Can you work these out from the drawing? Everything is in mm from the part's minimum corner. Round coordinates to 2 decimals unless told otherwise and drop trailing zeros. Loops run counter-clockwise (first coordinate to the right, second up) from the corner with the lowest first, then second, coordinate; pieces in that order, holes last. Notation, with made-up numbers: M -7.5,-25 L 16.5,-25 A18 ccw 16.5,-3 Z; hole C 78,-17.75 d9. An arc over 180 degrees is marked long. Return JSON: item names as keys, results as strings. Group by question number.
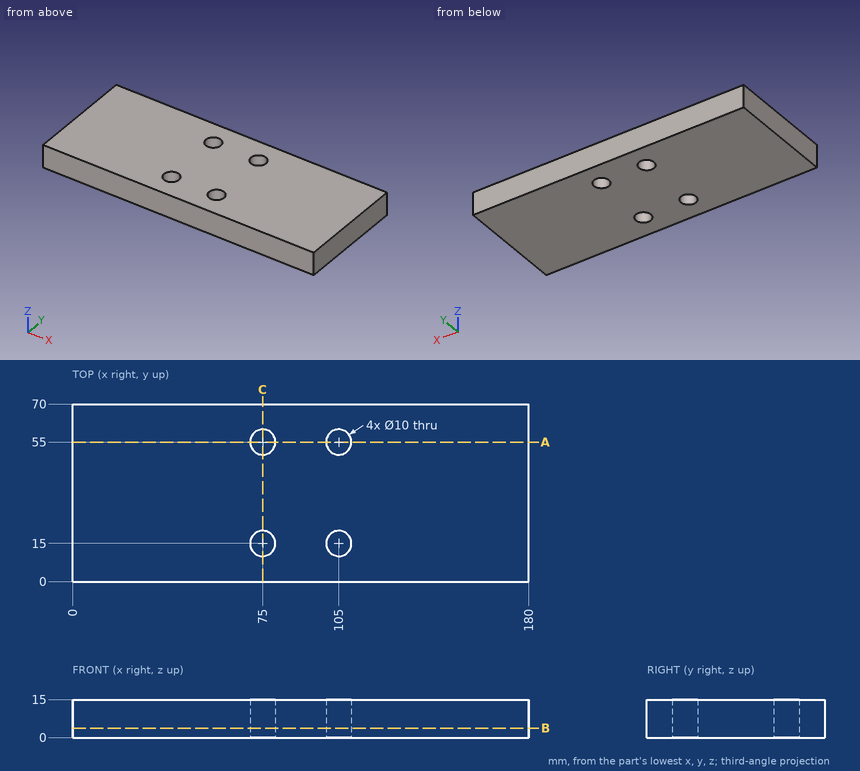
1. If we section it at B-B, the plane z = 3.75: Please give me the cut outline in (x, y), then the cut area to 3 significant figures.
2. If we section it at C-C, the plane x = 75: Please give me the cut outline in (y, z), then the cut area to 3 significant figures.
3. If we section it at A-A, the plane y = 55: Please give me the cut outline in (x, z), then the cut area to 3 significant figures.
4. I'm going to push a flat-ended pin straight in: pin 1 Ø4 at (x, y) = (130.5, 27) entering from -Z. Where does the tip first touch, or does it pass through?
5. I need wall thicknesses on probe 1 along Y at (x, z) = (105, 4.5); probe 2 along X at (y, z) = (54, 6.75). Which ranges of each line are inside material? Lowest first, please.
Geometry results:
{
 "1": {"outline": "M 0,0 L 180,0 L 180,70 L 0,70 Z; hole C 75,15 d10; hole C 75,55 d10; hole C 105,15 d10; hole C 105,55 d10", "area": "12,300 mm^2"},
 "2": {"outline": "M 0,0 L 10,0 L 10,15 L 0,15 Z; M 20,0 L 50,0 L 50,15 L 20,15 Z; M 60,0 L 70,0 L 70,15 L 60,15 Z", "area": "750 mm^2"},
 "3": {"outline": "M 0,0 L 70,0 L 70,15 L 0,15 Z; M 80,0 L 100,0 L 100,15 L 80,15 Z; M 110,0 L 180,0 L 180,15 L 110,15 Z", "area": "2,400 mm^2"},
 "4": {"pin 1": "z = 0"},
 "5": {"probe 1": "0 to 10, 20 to 50, 60 to 70", "probe 2": "0 to 70.1, 79.9 to 100.1, 109.9 to 180"}
}
